```python
from build123d import *
from OCP.BRepFilletAPI import BRepFilletAPI_MakeChamfer

# Parameters (mm, degrees)
BOSS_EXTRUDE3_DEPTH       = 100
BOSS_EXTRUDE4_START       = -25
BOSS_EXTRUDE4_DEPTH       = 135
FILLET2_R                 = 30
SKETCH8_R                 = 28
CUT_EXTRUDE2_DEPTH        = 85
CHAMFER2_SIZE             = 25
CHAMFER2_SIZE2            = 68.686935486
SKETCH9_R                 = 10
CUT_EXTRUDE3_DEPTH        = 858.264154976
FILLET2_OF_MIRROR1_R      = 30
CHAMFER2_OF_MIRROR1_SIZE  = 25
CHAMFER2_OF_MIRROR1_SIZE2 = 68.686935486
SKETCH10_R                = 55
CUT_EXTRUDE4_DEPTH        = 7
SKETCH11_R                = 55
CUT_EXTRUDE5_DEPTH        = 7


with BuildPart() as part:
    # Sweep3: sweep along a path in Sketch2
    with BuildLine(Plane(origin=(0, 0, 0), x_dir=(0, 0, -1), z_dir=(1, 0, 0))) as sweep3_path:
        Line((40, -707.115), (35.150009844, -667.615))
        ThreePointArc((35.150009844, -667.615), (21.699722473, -628.444195566), (-6.468256478, -598.082589677))
        Line((-6.468256478, -598.082589677), (-15.272697684, -591.87285015))
        ThreePointArc((-15.272697684, -591.87285015), (-77.559200743, -520.481595506), (-100, -428.434160824))
        Line((-100, -428.434160824), (-100, -372.115))
        Line((-100, -372.115), (-100, 0))
    # Sketch1 → Sweep3 (sweep)
    with BuildSketch(Plane(origin=(0, 0, 0), x_dir=(1, 0, 0), z_dir=(0, 1, 0))):
        Polygon((-45, 0), (-45, -20), (-12.5, -20), (-12.5, -80), (-45, -80), (-45, -100), (45, -100), (45, -80), (12.5, -80), (12.5, -20), (45, -20), (45, 0), align=None)
    sweep3 = sweep(path=sweep3_path.line)

    # Sketch6 → Boss-Extrude3 (add)
    with BuildSketch(Plane(origin=(0, 6.523203495, -53.127229086), x_dir=(-1, 0, 0), z_dir=(0, 0.12186934340514098, -0.992546151641323))):
        Polygon((-45, -706.719045754), (45, -706.719045754), (37.5, -731.719045754), (-37.5, -731.719045754), align=None)
    boss_extrude3 = extrude(amount=-BOSS_EXTRUDE3_DEPTH)

    # Sketch7 → Boss-Extrude4 (add)
    with BuildSketch(Plane(origin=(0, -726.264922946, -89.174119663), x_dir=(1, 0, 0), z_dir=(0, -0.992546151641323, -0.12186934340514098)).offset(BOSS_EXTRUDE4_START)):
        Polygon((-39.489238574, 37.473794696), (45, 31.565731599), (39.489238574, -47.241828371), (-45, -41.333765274), align=None)
    boss_extrude4 = extrude(amount=BOSS_EXTRUDE4_DEPTH)

    # Fillet2
    fillet2_edges = [part.edges().sort_by_distance(p)[0] for p in [
        (-42.244619287, -835.209793586, -104.495346909),
        (42.244619287, -834.489781816, -110.3593722),
    ]]
    fillet(fillet2_edges, radius=FILLET2_R)

    # Sketch8 → Cut-Extrude2 (cut)
    with BuildSketch(Plane(origin=(-3.095242597, 5.394428439, -43.934093987), x_dir=(-0.9975640426646005, -0.00837869546975235, 0.06925155770727769), z_dir=(-0.06975647374412558, 0.12157247580973782, -0.9901283591011198))):
        with Locations(Location((-0.444559855, -801.718997, 0), (0, 0, 89.992929705))):
            Circle(SKETCH8_R)
    cut_extrude2 = extrude(amount=-CUT_EXTRUDE2_DEPTH, mode=Mode.SUBTRACT)

    # Chamfer2: one chamfer whose edges measure the first distance from different faces: ONE call of the kernel's chamfer builder (chamfer() names one face for all edges)
    chamfer2_edges_1 = [part.edges().sort_by_distance(p)[0] for p in [
        (12.5, -701.02153283, -89.627307582),
    ]]
    chamfer2_side_1 = [part.faces().sort_by_distance(p)[0] for p in [
        (28.75, -701.02153283, -89.627307582),
    ]]
    chamfer2_edges_2 = [part.edges().sort_by_distance(p)[0] for p in [
        (-12.5, -701.02153283, -89.627307582),
    ]]
    chamfer2_side_2 = [part.faces().sort_by_distance(p)[0] for p in [
        (-28.75, -701.02153283, -89.627307582),
    ]]
    chamfer2 = BRepFilletAPI_MakeChamfer(part.part.solid().wrapped)
    for e in chamfer2_edges_1:
        chamfer2.Add(CHAMFER2_SIZE, CHAMFER2_SIZE2, e.wrapped, chamfer2_side_1[0].wrapped)  # the first distance lies on this face
    for e in chamfer2_edges_2:
        chamfer2.Add(CHAMFER2_SIZE, CHAMFER2_SIZE2, e.wrapped, chamfer2_side_2[0].wrapped)  # the first distance lies on this face
    add(Compound.cast(chamfer2.Shape()), mode=Mode.REPLACE)

    # Sketch9 → Cut-Extrude3 (cut, through all)
    with BuildSketch(Plane(origin=(-41.904757403, -0.357109604, 2.908424331), x_dir=(0.06923400560903198, 0.0005900076719097519, 0.9976002728339021), z_dir=(-0.9975640502598241, -0.008501175653454889, 0.06923651956680364))):
        with Locations(Location((-103.821376482, -766.779055644, 0), (0, 0, 359.966193827))):
            Circle(SKETCH9_R)
    cut_extrude3 = extrude(amount=-CUT_EXTRUDE3_DEPTH, mode=Mode.SUBTRACT)

    # Mirror1: Sweep3, Boss-Extrude3, Boss-Extrude4, Cut-Extrude2, Cut-Extrude3 across plane
    add(sweep3.mirror(Plane.ZX))
    add(boss_extrude3.mirror(Plane.ZX))
    add(boss_extrude4.mirror(Plane.ZX))
    add(cut_extrude2.mirror(Plane.ZX), mode=Mode.SUBTRACT)
    add(cut_extrude3.mirror(Plane.ZX), mode=Mode.SUBTRACT)

    # Fillet2 of Mirror1
    fillet2_of_mirror1_edges = [part.edges().sort_by_distance(p)[0] for p in [
        (-42.244619287, 835.209793586, -104.495346909),
        (42.244619287, 834.489781816, -110.3593722),
    ]]
    fillet(fillet2_of_mirror1_edges, radius=FILLET2_OF_MIRROR1_R)

    # Chamfer2 of Mirror1: one chamfer whose edges measure the first distance from different faces: ONE call of the kernel's chamfer builder (chamfer() names one face for all edges)
    chamfer2_of_mirror1_edges_1 = [part.edges().sort_by_distance(p)[0] for p in [
        (12.5, 701.02153283, -89.627307582),
    ]]
    chamfer2_of_mirror1_side_1 = [part.faces().sort_by_distance(p)[0] for p in [
        (28.75, 701.02153283, -89.627307582),
    ]]
    chamfer2_of_mirror1_edges_2 = [part.edges().sort_by_distance(p)[0] for p in [
        (-12.5, 701.02153283, -89.627307582),
    ]]
    chamfer2_of_mirror1_side_2 = [part.faces().sort_by_distance(p)[0] for p in [
        (-28.75, 701.02153283, -89.627307582),
    ]]
    chamfer2_of_mirror1 = BRepFilletAPI_MakeChamfer(part.part.solid().wrapped)
    for e in chamfer2_of_mirror1_edges_1:
        chamfer2_of_mirror1.Add(CHAMFER2_OF_MIRROR1_SIZE, CHAMFER2_OF_MIRROR1_SIZE2, e.wrapped, chamfer2_of_mirror1_side_1[0].wrapped)  # the first distance lies on this face
    for e in chamfer2_of_mirror1_edges_2:
        chamfer2_of_mirror1.Add(CHAMFER2_OF_MIRROR1_SIZE, CHAMFER2_OF_MIRROR1_SIZE2, e.wrapped, chamfer2_of_mirror1_side_2[0].wrapped)  # the first distance lies on this face
    add(Compound.cast(chamfer2_of_mirror1.Shape()), mode=Mode.REPLACE)

    # Sketch10 → Cut-Extrude4 (cut)
    with BuildSketch(Plane(origin=(2.415518829, 4.20979715, 34.286046382), x_dir=(0.9975640502598243, -0.008501175653454538, -0.06923651956680081), z_dir=(0.06975647374412557, 0.12157247580973786, 0.9901283591011197))):
        with Locations((0.345627789, 801.719045754)):
            Circle(SKETCH10_R)
    extrude(amount=-CUT_EXTRUDE4_DEPTH, mode=Mode.SUBTRACT)

    # Sketch11 → Cut-Extrude5 (cut)
    with BuildSketch(Plane(origin=(2.415518829, -4.20979715, 34.286046382), x_dir=(0.9975640502598243, 0.008501175653454538, -0.06923651956680081), z_dir=(0.06975647374412557, -0.12157247580973786, 0.9901283591011197))):
        with Locations((0.345627789, -801.719045754)):
            Circle(SKETCH11_R)
    extrude(amount=-CUT_EXTRUDE5_DEPTH, mode=Mode.SUBTRACT)


solid = part.part
```
Here's how the part is built. I have some questions about the finished solid (model axes, mm). A direction names the side the tool comes from. Give positions to 0.01 mm unless a question says otherwise; leave off trailing zeros. Loops run counter-clockwise (first coordinate to the right, second up) from the corner with the lowest first, then second, coordinate; pieces in that order, holes last. Notation, with made-up numbers: M 60.25,62 L 93.25,62 A21 cw 93.25,88 Z; hole C 43,85 d10. An arc over 180 degrees is marked long. Put each result on its own line as item: value. Start each with the question number.
(1) Will these pins go through, and if not, where does the flat tip stop? pin 1 Ø2 at (x, z) = (22.5, -11.5) entering from +Y; pin 2 Ø1.5 at (x, y) = (13, 135) entering from -Z; pin 3 Ø6 at (x, z) = (30, -112) entering from +Y.
(2) I want a section at B-B on z = 56. Please give me the cut outline in (x, y).
(3) For faces 1 (the flat face through (29, -6, 80)), 2 (the cylindrical face through (-1.08, 756.9, -104.85)), 3 (the flat face through (-29, -6, 20)), 4 (the cylindrical face through (-0.63, 578.09, -108.1)), which set-ups out of +Z, -Z, +X, -X, +Y, -Y let a thin tool reach every point of the face, with its end or its side?
(4) I need wall thicknesses on line 1 along Z through (x, y) = (-21, 58); line 2 along Y through (x, z) = (-14, -43.5); line 3 along Y through (x, z) = (-6.5, -107.5). Which ranges of each line are inside material? Lowest first, please. Write a range as [from, to].
(5) I want a section at A-A on y = -13.5. Please give me the cut outline in (x, z), then the cut area to 3 significant figures.
Answer block:
1. pin 1: y = 615.52
1. pin 2: z = 0
1. pin 3: y = 830.34
2. outline: M -45,-553.59 L 45,-553.59 L 45,-518.23 L 12.5,-518.23 L 12.5,518.23 L 45,518.23 L 45,553.59 L -45,553.59 L -45,518.23 L -12.5,518.23 L -12.5,-518.23 L -45,-518.23 Z
3. face 1: +X
3. face 2: none
3. face 3: -X
3. face 4: -Z, +X, -X
4. line 1: [0, 20], [80, 100]
4. line 2: [-731.87, -626.69], [-535.51, -510.95], [510.95, 535.51], [626.69, 731.87]
4. line 3: [-834.84, -822.01], [-757.84, -577.08], [577.08, 757.84], [822.01, 834.84]
5. outline: M -45,0 L 45,0 L 45,20 L 12.5,20 L 12.5,80 L 45,80 L 45,100 L -45,100 L -45,80 L -12.5,80 L -12.5,20 L -45,20 Z
5. area: 5,100 mm^2
